```python
from build123d import *

# Parameters (mm, degrees)
MODEL_R             = 1.300004804
MODEL_R_2           = 1.3
BOSS_EXTRUDE1_DEPTH = 3


with BuildPart() as part:
    # Model → Boss-Extrude1 (new body)
    with BuildSketch(Plane.XY):
        with BuildLine():
            ThreePointArc((63.8572156, 46.472930832), (65.173213816, 46.473407151), (65.83136885, 47.613005099))
            Line((65.83136885, 47.613005099), (68.83138654, 47.613005099))
            Line((68.83138654, 47.613005099), (68.83138654, 53.61311115))
            Line((68.83138654, 53.61311115), (71.231386535, 53.61311115))
            Line((71.231386535, 53.61311115), (71.231386535, 47.61311115))
            Line((71.231386535, 47.61311115), (74.231368849, 47.61311115))
            Line((74.231368849, 47.61311115), (74.231368849, 35.61311115))
            Line((74.231368849, 35.61311115), (71.231386533, 35.61311115))
            Line((71.231386533, 35.61311115), (71.231386533, 29.61311115))
            Line((71.231386533, 29.61311115), (68.831386538, 29.61311115))
            Line((68.831386538, 29.61311115), (68.831386538, 35.61293443))
            Line((68.831386538, 35.61293443), (65.831368849, 35.61293443))
            ThreePointArc((65.831368849, 35.61293443), (64.915944961, 39.030436678), (62.414363078, 41.532318088))
            Line((62.414363078, 41.532318088), (50.393576956, 48.333374046))
            ThreePointArc((50.393576956, 48.333374046), (50.904413755, 54.977754044), (56.710901802, 51.707672034))
            ThreePointArc((56.710901802, 51.707672034), (56.990071165, 50.734303435), (57.710211056, 50.022418261))
            Line((57.710211056, 50.022418261), (63.8572156, 46.472930832))
        make_face()
        with Locations((52.711979414, 51.613979963)):
            Circle(MODEL_R, mode=Mode.SUBTRACT)
        with Locations((70.031775439, 41.612672771)):
            Circle(MODEL_R_2, mode=Mode.SUBTRACT)
    extrude(amount=BOSS_EXTRUDE1_DEPTH)


solid = part.part
```
Here's how the part is built. I have some questions about the finished solid (model axes, mm). A direction names the side the tool comes from. Round coordinates to 2 decimals unless told otherwise and drop trailing zeros. Write each loop counter-clockwise with the first axis right and the second up, starting at its lowest first coordinate (ties: lowest second). Pieces come first, ordered by that corner, then holes.
Q1. Will these pins go through, and if not, where does the flat tip stop? P1, Ø1.5, axis at x = 62, z = 2.5, coming from the +Y side; P2, Ø1.5, axis at x = 67.5, z = 1.5, coming from the +Y side.
Q2. Please list where these lines run through material, in increasing order: probe 1 along Y at (x, z) = (71.5, 1.8); probe 2 along Y at (x, z) = (70, 2.6); probe 3 along X at (y, z) = (47, 1.5).
Q3. If we section it at D-D on x = 68: Write out the boundary of the cut face in (y, z).
Q4. If we section it at A-A on x = 52: Write out the boundary of the cut face in (y, z), plus the area to 3 significant figures.
Q5. If we mould it in two halves opening along X, with no side actions, what happens to faces 4 (the cylindrical face through (70.73, 42.71, 1.48)), 5 (the flat face through (71.231, 33, 1)), 6 (the flat face through (68.831, 33, 1))? For each: +X half, -X half, draft (parallel to the pull), parting line (faces both ways), or undercut.
Q6. If we section it at C-C on z = 1.9: Write out the boundary of the cut face in (x, y), plus the area to 3 significant figures.
Q7. Which directions (+Z, -Z, +X, -X, +Y, -Y) give clear straight access to the entire face, cutting with the end or side of a thin tool? Please do faces 1 (the flat face through (73, 47.613, 1)), 2 (the flat face through (67, 35.613, 1)), 3 (the flat face through (73, 35.613, 1)).
Q8. If we section it at B-B on y = 49.5: Write out the boundary of the cut face in (x, z).
Answer below:
1. P1: stops at y = 47.98
1. P2: stops at y = 47.61
2. probe 1: y = 35.61 to 47.61
2. probe 2: y = 29.61 to 40.31, 42.91 to 53.61
2. probe 3: x = 52.75 to 62.94, 65.68 to 74.23
3. outline: (35.61, 0) - (47.61, 0) - (47.61, 3) - (35.61, 3) - close
4. outline: (47.42, 0) - (50.53, 0) - (50.53, 3) - (47.42, 3) - close; (52.7, 0) - (55.37, 0) - (55.37, 3) - (52.7, 3) - close
4. area: 17.3 mm2
5. face 4: undercut
5. face 5: +X half
5. face 6: -X half
6. outline: (50.39, 48.33) - (62.41, 41.53) arc R6.83 cw to (65.83, 35.61) - (68.83, 35.61) - (68.83, 29.61) - (71.23, 29.61) - (71.23, 35.61) - (74.23, 35.61) - (74.23, 47.61) - (71.23, 47.61) - (71.23, 53.61) - (68.83, 53.61) - (68.83, 47.61) - (65.83, 47.61) arc R1.32 cw to (63.86, 46.47) - (57.71, 50.02) arc R2 cw to (56.71, 51.71) arc R3.95 ccw (long way) to start; hole circle Ø2.6 at (52.71, 51.61); hole circle Ø2.6 at (70.03, 41.61)
6. area: 235 mm2
7. face 1: +Z, -Z, +X, +Y
7. face 2: +Z, -Z, -X, -Y
7. face 3: +Z, -Z, +X, -Y
8. outline: (49.35, 0) - (58.61, 0) - (58.61, 3) - (49.35, 3) - close; (68.83, 0) - (71.23, 0) - (71.23, 3) - (68.83, 3) - close
